Part model, mm, in its own coordinate system. Face numbers are marked on the shaded views. A direction names the side the tool comes from. Round coordinates to 2 decimals unless told otherwise and drop trailing zeros. Loops run counter-clockwise (first coordinate to the right, second up) from the corner with the lowest first, then second, coordinate; pieces in that order, holes last.
(1) Probe probe 1 along Z at (x, y) = (0, 8); probe 2 along X at (y, z) = (3, 4); probe 3 along Z at (x, y) = (-5.5, 48.5). List the from-to ranges inside material, lowest first.
(2) Cut at B-B on y = 18.5. List the corners of the cut face in (x, z), then the cut area to 3 significant figures.
(3) Mould opens along X. For the marked faces 3, 4, 5 and 6 say: +X half, -X half, draft (parallel to the pull), parting line (faces both ways), or undercut.
(4) Tool access for the marked faces 1 and 2: list every direction of +Z, -Z, +X, -X, +Y, -Y with a clear straight run to the whole face (end or side of a thin tool).
(5) Cut at A-A on z = 0. List the corners of the cut face in (x, y).
(6) Cut at C-C on x = -12. List the corners of the cut face in (y, z), then the cut area to 3 significant figures.
(7) Cut at D-D on z = 28. List the corners of the cut face in (x, y).
(8) Flat gauge pins, fed straight in: pin 1 (8 mm diameter, centred on x = -39.5, y = 26.5, fed in from -Z); pin 2 (9 mm diameter, centred on x = -56.5, y = 33, fed in from -Z); pin 3 (10 mm diameter, centred on x = 46.5, y = 8, fed in from -Z). Where does each tip first touch, or does it go through?
from build123d import *

# Parameters (mm, degrees)
SKETCH2_R           = 90
BOSS_EXTRUDE1_DEPTH = 55
CUT_EXTRUDE1_DEPTH  = 30
SKETCH4_W           = 15
SKETCH4_H           = 40
CUT_EXTRUDE2_DEPTH  = 131.766968306
BOSS_EXTRUDE2_DEPTH = 43


with BuildPart() as part:
    # Sketch2 → Boss-Extrude1 (new body)
    with BuildSketch(Plane(origin=(0, 0, 0), x_dir=(1, 0, 0), z_dir=(0, 1, 0))):
        with Locations(Location((0, 0, 0), (0, 0, 270))):
            Circle(SKETCH2_R)
    extrude(amount=BOSS_EXTRUDE1_DEPTH)

    # Sketch3 → Cut-Extrude1 (cut)
    with BuildSketch(Plane(origin=(0, 55, 0), x_dir=(1, 0, 0), z_dir=(0, 1, 0))):
        with BuildLine():
            Line((-144.325071801, 37.5), (0, 37.5))
            ThreePointArc((0, 37.5), (37.5, 0), (0, -37.5))
            Line((0, -37.5), (-144.325071801, -37.5))
            ThreePointArc((-144.325071801, -37.5), (-181.825071801, 0), (-144.325071801, 37.5))
        make_face()
    extrude(amount=-CUT_EXTRUDE1_DEPTH, mode=Mode.SUBTRACT)

    # Sketch4 → Cut-Extrude2 (cut, through all)
    with BuildSketch(Plane(origin=(0, 25, 0), x_dir=(1, 0, 0), z_dir=(0, 1, 0))):
        Rectangle(SKETCH4_W, SKETCH4_H)
    extrude(amount=-CUT_EXTRUDE2_DEPTH, mode=Mode.SUBTRACT)

    # Sketch6_4 → Boss-Extrude2 (add)
    with BuildSketch(Plane(origin=(50, 0, 0), x_dir=(0, 0, -1), z_dir=(1, 0, 0))):
        with BuildLine():
            Line((-25, 33.917885912), (25, 33.917885912))
            ThreePointArc((25, 33.917885912), (30.997040934, 27.920844978), (25, 21.923804044))
            Line((25, 21.923804044), (-25, 21.923804044))
            ThreePointArc((-25, 21.923804044), (-30.997040934, 27.920844978), (-25, 33.917885912))
        make_face()
    extrude(amount=BOSS_EXTRUDE2_DEPTH)


solid = part.part
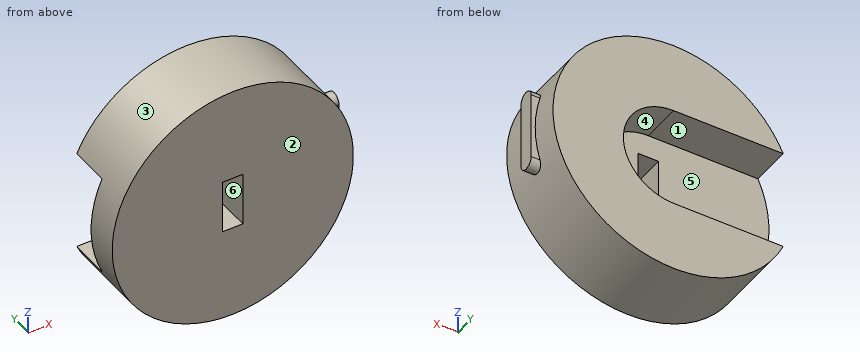
Final values:
1. probe 1: z = -90 to -20, 20 to 90
1. probe 2: x = -89.91 to -7.5, 7.5 to 89.91
1. probe 3: z = -89.83 to -37.5, 37.5 to 89.83
2. outline: circle Ø180 at (0, 0); hole (-7.5, -20) - (7.5, -20) - (7.5, 20) - (-7.5, 20) - close
2. area: 24,800 mm2
3. face 3: parting line
3. face 4: -X half
3. face 5: draft
3. face 6: undercut
4. face 1: -X, +Y
4. face 2: +Z, -Z, +X, -X, -Y
5. outline: (-90, 0) - (-7.5, 0) - (-7.5, 25) - (-90, 25) - close; (7.5, 0) - (90, 0) - (90, 21.92) - (93, 21.92) - (93, 33.92) - (90, 33.92) - (90, 55) - (37.5, 55) - (37.5, 25) - (7.5, 25) - close
6. outline: (0, -89.2) - (55, -89.2) - (55, -37.5) - (25, -37.5) - (25, 37.5) - (55, 37.5) - (55, 89.2) - (0, 89.2) - close
6. area: 7,560 mm2
7. outline: (-85.53, 0) - (85.53, 0) - (85.53, 22.73) - (93, 22.73) - (93, 33.11) - (85.53, 33.11) - (85.53, 55) - (24.94, 55) - (24.94, 25) - (-85.53, 25) - close
8. pin 1: stops at z = -82.7
8. pin 2: stops at z = -73.46
8. pin 3: stops at z = -79.86
